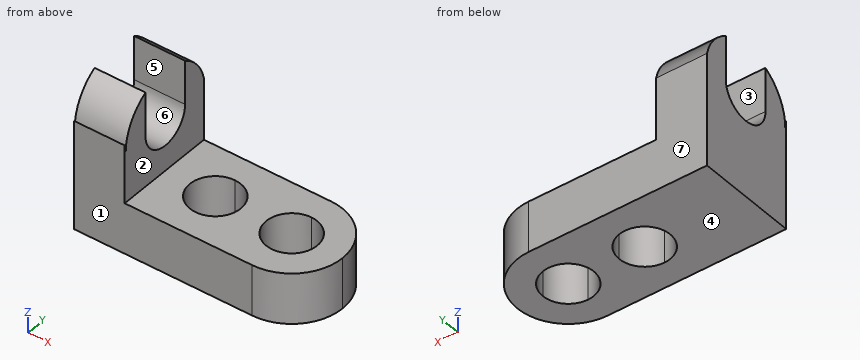
```python
from build123d import *

# Parameters (mm, degrees)
F1_DEPTH = 25.4
F3_DEPTH = 25.4
F5_DEPTH = 25.4


# Not quite as in the source:
# - a feature names something its author has since deleted; it is built from what else it names


with BuildPart() as f1:
    # F0 (on Front) → F1 (new body)
    with BuildSketch(Plane.XZ):
        Polygon((0, 38.1), (0, 0), (57.15, 0), (57.15, 12.7), (12.7, 12.7), (12.7, 38.1), align=None)
    extrude(amount=F1_DEPTH)

    # F2 (on Top) → F3 (cut)
    with BuildSketch(Plane.XY):
        with BuildLine():
            Line((25.4, -19.05), (25.4, -6.35))
            ThreePointArc((25.4, -6.35), (19.05, -12.7), (25.4, -19.05))
        make_face()
        with BuildLine():
            ThreePointArc((25.4, -19.05), (29.8901280605, -17.1901280605), (31.75, -12.7))
            ThreePointArc((31.75, -12.7), (29.8901280605, -8.2098719395), (25.4, -6.35))
            Line((25.4, -6.35), (25.4, -19.05))
        make_face()
        with BuildLine():
            Line((44.45, -19.05), (44.45, -6.35))
            ThreePointArc((44.45, -6.35), (38.1, -12.7), (44.45, -19.05))
        make_face()
        with BuildLine():
            ThreePointArc((50.8, -12.7), (48.9401280605, -8.2098719395), (44.45, -6.35))
            Line((44.45, -6.35), (44.45, -19.05))
            ThreePointArc((44.45, -19.05), (48.9401280605, -17.1901280605), (50.8, -12.7))
        make_face()
        with BuildLine():
            Line((57.15, -25.4), (57.15, -12.7))
            ThreePointArc((57.15, -12.7), (53.4302561211, -21.6802561211), (44.45, -25.4))
            Line((44.45, -25.4), (57.15, -25.4))
        make_face()
        with BuildLine():
            Line((57.15, 0), (44.45, 0))
            ThreePointArc((44.45, 0), (53.4302561211, -3.7197438789), (57.15, -12.7))
            Line((57.15, -12.7), (57.15, 0))
        make_face()
    extrude(amount=F3_DEPTH, mode=Mode.SUBTRACT)

    # F4 (on Right) → F5 (cut)
    with BuildSketch(Plane.YZ):
        with BuildLine():
            ThreePointArc((-18.7333624887, 25.4), (-12.3833624887, 19.05), (-6.0333624887, 25.4))
            ThreePointArc((-6.0333624887, 25.4), (-12.3833624887, 31.75), (-18.7333624887, 25.4))
        make_face()
        with BuildLine():
            ThreePointArc((-18.7333624887, 25.4), (-12.3833624887, 31.75), (-6.0333624887, 25.4))
            Line((-6.0333624887, 25.4), (-6.0333624887, 36.3985226281))
            ThreePointArc((-6.0333624887, 36.3985226281), (-9.0963606159, 37.6672579939), (-12.3833624887, 38.1))
            ThreePointArc((-12.3833624887, 38.1), (-15.6703643615, 37.6672579939), (-18.7333624887, 36.3985226281))
            Line((-18.7333624887, 36.3985226281), (-18.7333624887, 25.4))
        make_face()
        with BuildLine():
            ThreePointArc((-12.3833624887, 38.1), (-9.0963606159, 37.6672579939), (-6.0333624887, 36.3985226281))
            Line((-6.0333624887, 36.3985226281), (-6.0333624887, 38.1))
            Line((-6.0333624887, 38.1), (-12.3833624887, 38.1))
        make_face()
        with BuildLine():
            Line((-6.0333624887, 38.1), (-6.0333624887, 36.3985226281))
            ThreePointArc((-6.0333624887, 36.3985226281), (-1.3848398607, 31.75), (0.3166375113, 25.4))
            Line((0.3166375113, 25.4), (0.3166375113, 40.4268426491))
            Line((0.3166375113, 40.4268426491), (-27.6233624887, 40.4268426491))
            Line((-27.6233624887, 40.4268426491), (-25.0833624887, 25.4))
            ThreePointArc((-25.0833624887, 25.4), (-23.3818851168, 31.75), (-18.7333624887, 36.3985226281))
            Line((-18.7333624887, 36.3985226281), (-18.7333624887, 38.1))
            Line((-18.7333624887, 38.1), (-12.3833624887, 38.1))
            Line((-12.3833624887, 38.1), (-6.0333624887, 38.1))
        make_face()
        with BuildLine():
            Line((-18.7333624887, 38.1), (-18.7333624887, 36.3985226281))
            ThreePointArc((-18.7333624887, 36.3985226281), (-15.6703643615, 37.6672579939), (-12.3833624887, 38.1))
            Line((-12.3833624887, 38.1), (-18.7333624887, 38.1))
        make_face()
    extrude(amount=F5_DEPTH, mode=Mode.SUBTRACT)


solid = f1.part
```
Model file for the job. Use its own axes, mm. Face numbers are marked on the shaded views. A direction names the side the tool comes from. Coordinates: 2 decimals unless noted, no trailing zeros. Order: outer loops, then holes, each group sorted by start corner. A loop starts at its lowest first (then second) coordinate and runs counter-clockwise, first axis right, second up. Notation, with made-up numbers: (-2, -5) -> (18, -5) arc R21 cw to (18, 25) -> close; hole circle Ø11 at (23.25, 62.25). An arc over 180 degrees is marked (long way). Answer as a JSON object with one key per item and string values. Group by question number.
1) Cut at A-A, the plane x = 47. Write the cut outline in (y, z), then the cut area to 3 significant figures.
2) Flat gauge pins, fed straight in: pin 1 (1.5 mm diameter, centred on x = 20, z = 15, fed in from -Y); pin 2 (1.5 mm diameter, centred on x = 32.5, y = -6.5, fed in from -Z). Where does each tip first touch, or does it go through?
3) Which spindle directions (+Z, -Z, +X, -X, +Y, -Y) get a long thin tool onto all of the face, cutting with end or side? Do the marked faces 1, 2 and 3. Say none if no direction does.
4) Cut at B-B, the plane y = -14.25. Write the cut outline in (x, z), then the cut area to 3 significant figures.
5) Cut at C-C, the plane x = 12. Write the cut outline in (y, z).
6) Pull direction Y, two halves, no side cores. Call the marked faces 4, 5, 6 and 7: +Y half, -Y half, draft (parallel to the pull), parting line (faces both ways), or undercut.
7) Cut at D-D, the plane z = 14.5. Write the cut outline in (x, y).
8) Drill centre lines: L1, parallel to X at y = -12.75, z = 11.5; L2, parallel to X at y = -8.5, z = 5.5; L3, parallel to Z at x = 34, y = -19. Where is each one in solid material? Low to high.
Check values:
{
 "1": {"outline": "(-25.14, 0) -> (-18.52, 0) -> (-18.52, 12.7) -> (-25.14, 12.7) -> close; (-6.88, 0) -> (-0.26, 0) -> (-0.26, 12.7) -> (-6.88, 12.7) -> close", "area": "168 mm²"},
 "2": {"pin 1": "passes through", "pin 2": "stops at z = 0"},
 "3": {"face 1": "+Z, -Z, +X, -X, -Y", "face 2": "+Z, +X, +Y, -Y", "face 3": "+Z, +X, -X"},
 "4": {"outline": "(0, 0) -> (19.24, 0) -> (19.24, 12.7) -> (12.7, 12.7) -> (12.7, 19.33) -> (0, 19.33) -> close; (31.56, 0) -> (38.29, 0) -> (38.29, 12.7) -> (31.56, 12.7) -> close; (50.61, 0) -> (57.06, 0) -> (57.06, 12.7) -> (50.61, 12.7) -> close", "area": "496 mm²"},
 "5": {"outline": "(-25.4, 0) -> (0, 0) -> (0, 28.22) arc R12.7 ccw to (-6.03, 36.4) -> (-6.03, 25.4) arc R6.35 cw to (-18.73, 25.4) -> (-18.73, 36.4) arc R12.7 ccw to (-25.08, 25.4) -> (-25.4, 27.27) -> close"},
 "6": {"face 4": "draft", "face 5": "undercut", "face 6": "undercut", "face 7": "+Y half"},
 "7": {"outline": "(0, -25.4) -> (12.7, -25.4) -> (12.7, 0) -> (0, 0) -> close"},
 "8": {"L1": "x = 0 to 19.05, 31.75 to 38.1, 50.8 to 57.15", "L2": "x = 0 to 20.64, 30.16 to 39.69, 49.21 to 56.44", "L3": "z = 0 to 12.7"}
}
